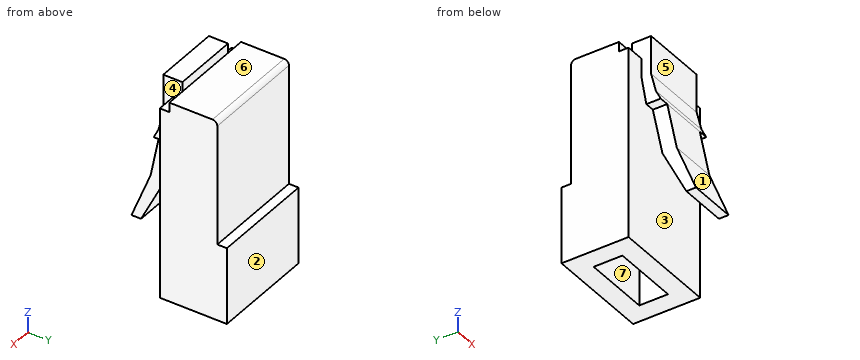
from build123d import *

# Parameters (mm, degrees)
SKETCH_2_W          = 11
SKETCH_2_H          = 6
EXTRUDE_1_DEPTH     = 5
SKETCH_3_W          = 11
SKETCH_3_H          = 6
EXTRUDE_2_DEPTH     = 8
SKETCH_4_W          = 11
SKETCH_4_H          = 7
EXTRUDE_3_DEPTH     = 8
SKETCH_6_W          = 7
SKETCH_6_H          = 2
EXTRUDE_4_DEPTH     = 1
SKETCH_8_W          = 2
SKETCH_8_H          = 1
CUT_EXTRUDE_1_DEPTH = 1
SKETCH_10_W         = 7
SKETCH_10_H         = 3
EXTRUDE_5_DEPTH     = 1
EXTRUDE_6_DEPTH     = 7
EXTRUDE_7_DEPTH     = 5
SKETCH_14_W         = 7
SKETCH_14_H         = 3
CUT_EXTRUDE_2_DEPTH = 8
FILLET_1_R          = 0.5


with BuildPart() as part:
    # Эскиз2 → Бобышка-Вытянуть1 (new body)
    with BuildSketch(Plane.XY):
        with Locations((5.5, 3)):
            Rectangle(SKETCH_2_W, SKETCH_2_H)
    extrude(amount=EXTRUDE_1_DEPTH)

    # Эскиз3 → Бобышка-Вытянуть2 (add)
    with BuildSketch(Plane(origin=(0, 0, 0), x_dir=(-1, 0, 0), z_dir=(0, 0, -1))):
        with Locations((-5.5, 3)):
            Rectangle(SKETCH_3_W, SKETCH_3_H)
    extrude(amount=EXTRUDE_2_DEPTH)

    # Эскиз4 → Бобышка-Вытянуть3 (add)
    with BuildSketch(Plane(origin=(0, 0, -8), x_dir=(-1, 0, 0), z_dir=(0, 0, -1))):
        with Locations((-5.5, 3.5)):
            Rectangle(SKETCH_4_W, SKETCH_4_H)
    extrude(amount=EXTRUDE_3_DEPTH)

    # Эскиз6 → Бобышка-Вытянуть4 (add)
    with BuildSketch(Plane.XY.offset(5)):
        with Locations((5.5, 0)):
            Rectangle(SKETCH_6_W, SKETCH_6_H)
    extrude(amount=EXTRUDE_4_DEPTH)

    # Эскиз8 → Вырез-Вытянуть1 (cut)
    with BuildSketch(Plane.XY.offset(5)):
        with Locations((1, 0.5)):
            Rectangle(SKETCH_8_W, SKETCH_8_H)
        with Locations((10, 0.5)):
            Rectangle(SKETCH_8_W, SKETCH_8_H)
    extrude(amount=-CUT_EXTRUDE_1_DEPTH, mode=Mode.SUBTRACT)

    # Эскиз10 → Бобышка-Вытянуть5 (add)
    with BuildSketch(Plane.XZ):
        with Locations((5.5, 3.5)):
            Rectangle(SKETCH_10_W, SKETCH_10_H)
    extrude(amount=EXTRUDE_5_DEPTH)

    # Эскиз12 → Бобышка-Вытянуть6 (add)
    with BuildSketch(Plane(origin=(9, 0, 0), x_dir=(0, 0, -1), z_dir=(1, 0, 0))):
        Polygon((-2, 0), (1, -0.5), (1, -2), (0, -1.5), (-2, -1), align=None)
    extrude(amount=-EXTRUDE_6_DEPTH)

    # Эскиз13 → Бобышка-Вытянуть7 (add)
    with BuildSketch(Plane(origin=(8, 0, 0), x_dir=(0, 0, -1), z_dir=(1, 0, 0))):
        Polygon((1, -0.5), (6, -1.5), (11, -4), (11, -5), (6, -3), (1, -2), align=None)
    extrude(amount=-EXTRUDE_7_DEPTH)

    # Эскиз14 → Вырез-Вытянуть2 (cut)
    with BuildSketch(Plane(origin=(0, 0, -16), x_dir=(-1, 0, 0), z_dir=(0, 0, -1))):
        with Locations((-5.5, 3.5)):
            Rectangle(SKETCH_14_W, SKETCH_14_H)
    extrude(amount=-CUT_EXTRUDE_2_DEPTH, mode=Mode.SUBTRACT)

    # Скругление1
    fillet_1_edges = [part.edges().sort_by_distance(p)[0] for p in [
        (5.5, 6, 5),
    ]]
    fillet(fillet_1_edges, radius=FILLET_1_R)


solid = part.part
Geometry check sheet. Reference: the model listing, model coordinates, mm. Face numbers are marked on the shaded views. A direction names the side the tool comes from. Coordinates: 2 decimals unless noted, no trailing zeros. Write each loop counter-clockwise with the first axis right and the second up, starting at its lowest first coordinate (ties: lowest second). Pieces come first, ordered by that corner, then holes. Notation, with made-up numbers: (57.5, 82) -> (109.5, 82) arc R25 cw to (109.5, 99) -> close; hole circle Ø5 at (59, 83.25). An arc over 180 degrees is marked (long way). One line per question, with ' | ' between items.
1. Thickness scan on probe 1 along X at (y, z) = (3.75, -13); probe 2 along Y at (x, z) = (8.25, -9); probe 3 along Y at (x, z) = (10.5, -2). Record the ranges inside material, lowest first. Write a range as from..to.
Answers:
probe 1: x = 0..2, 9..11 | probe 2: y = 0..2, 5..7 | probe 3: y = 0..6
2. Set-up check for the marked faces 5, 6 and 7: record each of +Z, -Z, +X, -X, +Y, -Y from which the full face is reachable in a straight line by a thin tool's end or side.
Answers:
face 5: +Z, +X, -X, -Y | face 6: +Z, +X, -X, +Y | face 7: -Z
3. Cross-section at A-A on z = -10. Record the cut outline in (x, y).
Answers:
outline: (0, 0) -> (11, 0) -> (11, 7) -> (0, 7) -> close; (3, -4.6) -> (8, -4.6) -> (8, -3.5) -> (3, -3.5) -> close; hole (2, 2) -> (9, 2) -> (9, 5) -> (2, 5) -> close
4. Cross-section at B-B on z = -3. Record the cut outline in (x, y), and give its area (3 significant figures).
Answers:
outline: (0, 0) -> (11, 0) -> (11, 6) -> (0, 6) -> close; (3, -2.4) -> (8, -2.4) -> (8, -0.9) -> (3, -0.9) -> close | area: 73.5 mm²
5. Draft check along Y on the marked faces 1, 2, 3 and 4. Enter one of: +Y half, -Y half, draft (parallel to the pull), parting line (faces both ways), or undercut.
Answers:
face 1: -Y half | face 2: +Y half | face 3: undercut | face 4: draft
6. Cross-section at C-C on y = -1.75. Record the cut outline in (x, z), and give its area (3 significant figures).
Answers:
outline: (2, -1) -> (3, -1) -> (3, -6.5) -> (8, -6.5) -> (8, -1) -> (9, -1) -> (9, -0.5) -> (2, -0.5) -> close | area: 31.0 mm²
7. Depth check by flat-ended pin: pin 1 Ø1.5 at (y, z) = (5.5, -6) entering from -X; pin 2 Ø5.5 at (x, z) = (7.5, -3) entering from -Y; pin 3 Ø1.5 at (y, z) = (-2.5, -5) entering from +X; pin 4 Ø0.9 at (y, z) = (-0.5, 2.5) entering from +X. Enter the tip coordinate at first touch or a pass-through.
Answers:
pin 1: stops at x = 0 | pin 2: stops at y = -2.95 | pin 3: stops at x = 8 | pin 4: stops at x = 9
8. Cross-section at D-D on x = 9.25. Record the cut outline in (y, z).
Answers:
outline: (0, -16) -> (7, -16) -> (7, -8) -> (6, -8) -> (6, 4.5) arc R0.5 ccw to (5.5, 5) -> (1, 5) -> (1, 4) -> (0, 4) -> close
